Geometry check sheet. Reference: the model listing, model coordinates, mm. A direction names the side the tool comes from. Coordinates: 2 decimals unless noted, no trailing zeros. Write each loop counter-clockwise with the first axis right and the second up, starting at its lowest first coordinate (ties: lowest second). Pieces come first, ordered by that corner, then holes. Notation, with made-up numbers: (55.5, -31.5) -> (103.5, -31.5) arc R37 ccw to (103.5, 7.5) -> close; hole circle Ø11 at (-3, 57). An arc over 180 degrees is marked (long way). Answer in a Markdown table with one row per item. Add a question column.
1. Set-up check for faces 1 (the flat face through (80, 2, -75)), 2 (the cylindrical face through (68.594, 2.465, -37.028)), 3 (the cylindrical face through (62.747, 2.465, -12.621)): record each of +Z, -Z, +X, -X, +Y, -Y from which the full face is reachable in a straight line by a thin tool's end or side.
2. Mould release check, pull along Z, two halves, no side actions. Record for faces 4 (the cylindrical face through (-7.142, 2.465, -22.727)), 5 (the flat face through (-8, 2, -60)), 6 (the flat face through (59, 5, -23)), 7 (the cylindrical face through (42.747, 2.465, -12.621)): pulls with the +Z half, pulls with the -Z half, needs draft (parallel to the pull), parting line crosses it, or undercut.
3. Depth check by flat-ended pin: P1, Ø2.5, axis at x = -9.5, y = 3.5, coming from the -Z side. Enter the tip coordinate at first touch or a pass-through.
4. Cross-section at C-C on z = -52.5. Record the cut outline in (x, y).
5. Cross-section at B-B on y = 1.85. Give the number of separate pieces and of enclosed holes in the cut face, and give its area (3 significant figures).
6. Cross-section at D-D on x = 20. Record the cut outline in (y, z), and give its area (3 significant figures).
7. Cross-section at A-A on x = -7.5. Record the cut outline in (y, z), and give its area (3 significant figures).
8. Scan lines: L1, parallel to Z at x = 92.5, y = 2.5; L2, parallel to Z at x = 40, y = 3.35; L3, parallel to X at y = 2.1, z = -78. Record each from-to range of solid material in increasing order. Write a range as from..to.
Autodesk Inventor part; units mm, degrees
ref_plane "YZ Plane" through (0, 0, 0) normal (1, 0, 0) x (0, 1, 0)
ref_plane "XZ Plane" through (0, 0, 0) normal (0, 1, 0) x (-1, 0, 0)
ref_plane "XY Plane" through (0, 0, 0) normal (0, 0, 1) x (1, 0, 0)
sketch "Sketch1" plane through (0, 0, 0) normal (0, 1, 0) x (-1, 0, 0)
  line L0 (0, 0) -> (15, 0)
  line L1 (15, 0) -> (15, -60)
  line L2 (15, -60) -> (0, -60)
  line L3 (0, -60) -> (0, 0)
  circle A0 centre (7.5, -40) radius 2.75
  line L4 (0, 0) -> (-105, 0)
  line L5 (-105, 0) -> (-105, -25)
  line L6 (-105, -25) -> (0, -25)
  line L7 (0, -25) -> (0, 0)
  line L8 (-105, -25) -> (-80, -25)
  line L9 (-80, -25) -> (-80, -85)
  line L10 (-80, -85) -> (-105, -85)
  line L11 (-105, -85) -> (-105, -25)
  circle A1 centre (7.5, -20) radius 2.75
  circle A2 centre (-20, -12.5) radius 2.75
  circle A3 centre (-40, -12.5) radius 2.75
  circle A4 centre (-60, -12.5) radius 2.75
  circle A5 centre (-80, -12.5) radius 2.75
  circle A6 centre (-92.5, -45) radius 2.75
  circle A7 centre (-92.5, -65) radius 2.75
  line L12 (-30, -25) -> (-30, 0)
  dimension "d0" = 15
  dimension "d1" = 60
  dimension "d2" = 5.5
  dimension "d3" = 40
  dimension "d4" = 7.5
  dimension "d5" = 105
  dimension "d6" = 25
  dimension "d7" = 60
  dimension "d8" = 25
  dimension "d9" = 5.5
  dimension "d10" = 7.5
  dimension "d11" = 20
  dimension "d12" = 5.5
  dimension "d13" = 12.5
  dimension "d14" = 20
  dimension "d17" = 20
  dimension "d22" = 5.5
  dimension "d23" = 5.5
  dimension "d24" = 12.5
  dimension "d25" = 12.5
  dimension "d26" = 20
  dimension "d27" = 20
  dimension "d31" = 10
extrude "Extrusion1" add sketch "Sketch1" along normal blind 5
fillet "Fillet1" radius 40 2 edges at (80, 2.5, -25) (0, 2.5, -25)
properties part number "Brace" material "Aluminum 6061"
Results found:
| question | item | result |
|---|---|---|
| 1 | face 1 | -Z, -X, +Y, -Y |
| 1 | face 2 | -Z, +Y, -Y |
| 1 | face 3 | +Y, -Y |
| 2 | face 4 | undercut |
| 2 | face 5 | pulls with the -Z half |
| 2 | face 6 | needs draft |
| 2 | face 7 | undercut |
| 3 | P1 | stops at z = -60 |
| 4 | outline | (-15, 0) -> (1.69, 0) -> (1.69, 5) -> (-15, 5) -> close; (78, 0) -> (105, 0) -> (105, 5) -> (78, 5) -> close |
| 5 | separate pieces | 1 |
| 5 | enclosed holes | 8 |
| 5 | area | 5,510 mm^2 |
| 6 | outline | (0, -30.18) -> (5, -30.18) -> (5, -15.25) -> (0, -15.25) -> close; (0, -9.75) -> (5, -9.75) -> (5, 0) -> (0, 0) -> close |
| 6 | area | 123 mm^2 |
| 7 | outline | (0, -60) -> (5, -60) -> (5, -42.75) -> (0, -42.75) -> close; (0, -37.25) -> (5, -37.25) -> (5, -22.75) -> (0, -22.75) -> close; (0, -17.25) -> (5, -17.25) -> (5, 0) -> (0, 0) -> close |
| 7 | area | 245 mm^2 |
| 8 | L1 | z = -85..-67.75, -62.25..-47.75, -42.25..0 |
| 8 | L2 | z = -25..-15.25, -9.75..0 |
| 8 | L3 | x = 80..105 |
